Autodesk Inventor part; units mm, degrees
ref_plane "YZ Plane" through (0, 0, 0) normal (1, 0, 0) x (0, 1, 0)
ref_plane "XZ Plane" through (0, 0, 0) normal (0, 1, 0) x (-1, 0, 0)
ref_plane "XY Plane" through (0, 0, 0) normal (0, 0, 1) x (1, 0, 0)
sketch "Sketch1" plane through (0, 0, 0) normal (0, 0, 1) x (1, 0, 0)
  line L0 (-4.2, 0) -> (4.2, 0)
  line L1 (0, -1.5) -> (0, 9)
  line L2 (-3, 7.5) -> (3, 7.5)
  line L3 (3, 7.5) -> (3, 0)
  line L4 (3, 0) -> (-3, 0)
  line L5 (-3, 0) -> (-3, 7.5)
  point P0 (0, 0)
  point P1 (0, 0)
  dimension "d0" = 6
  dimension "d1" = 7.5
extrude "Extrusion1" add sketch "Sketch1" along normal mid plane 9.8
fillet "Fillet1" radius 3 2 edges at (3, 7.5, 0) (-3, 7.5, 0)
mirror "Mirror1" about plane through (-3, 0, 0) normal (0, -1, 0)
sketch "Sketch2" plane through (3, 4.5, 4.9) normal (1, 0, 0) x (0, 0, -1)
  point P0 (4.9, -4.5)
hole "Hole1" at (3, 0, 0) direction (-1, 0, 0) diameter 5 end through all
fillet "Fillet2" radius 2 2 edges at (3, 0, 2.5) (-3, 0, 2.5)
properties part number "P103" material "ABS Plastic"
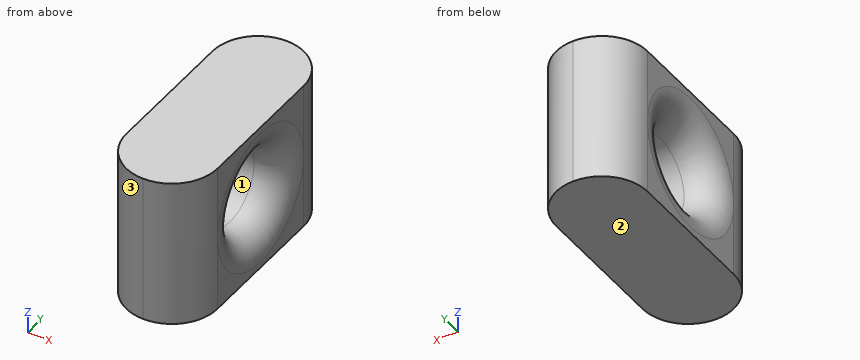
The model under review builds one solid part; all positions refer to its coordinate system, in mm. Face numbers are marked on the shaded views. Round coordinates to 2 decimals unless told otherwise and drop trailing zeros. Order: outer loops, then holes, each group sorted by start corner. A loop starts at its lowest first (then second) coordinate and runs counter-clockwise, first axis right, second up. Notation, with made-up numbers: M 23,19 L 43,19 A20 ccw 43,51 Z; hole C 65,80.25 d11. An arc over 180 degrees is marked long. Use a Markdown table: item, result.
1) Consider section C-C (x = -0.5). Write out the cut boundary in (y, z), then the cut area to 3 significant figures.
Report:
| item | result |
|---|---|
| outline | M -7.46,-4.9 L 7.46,-4.9 L 7.46,4.9 L -7.46,4.9 Z; hole C 0,0 d5 |
| area | 127 mm^2 |
2) Consider section B-B (y = 0). Write out the cut boundary in (x, z).
Report:
| item | result |
|---|---|
| outline | M -3,-4.9 L 3,-4.9 L 3,-4.5 A2 ccw 1,-2.5 L -1,-2.5 A2 ccw -3,-4.5 Z; M -3,4.5 A2 ccw -1,2.5 L 1,2.5 A2 ccw 3,4.5 L 3,4.9 L -3,4.9 Z |
3) Wall thickness on line 1 along Z through (x, y) = (-0.25, 0); line 2 along Y through (x, z) = (-0.4, 0); line 3 along Y through (x, z) = (-2.25, -0.25): over which ranges is each line inside the solid? List them lowest first. Write a range as [from, to].
Report:
| item | result |
|---|---|
| line 1 | [-4.9, -2.5], [2.5, 4.9] |
| line 2 | [-7.47, -2.5], [2.5, 7.47] |
| line 3 | [-6.48, -2.93], [2.93, 6.48] |
4) Consider section D-D (y = 6). Write out the cut boundary in (x, z), then the cut area to 3 significant figures.
Report:
| item | result |
|---|---|
| outline | M -2.6,-4.9 L 2.6,-4.9 L 2.6,4.9 L -2.6,4.9 Z |
| area | 50.9 mm^2 |
5) Draft analysis for pull direction Z (two halves, no side actions). For the marked faces 1, 2 and 3, state which applies: released by +Z, released by -Z, zero draft, split by the parting line, or undercut.
Report:
| item | result |
|---|---|
| face 1 | undercut |
| face 2 | released by -Z |
| face 3 | zero draft |
6) Insertion check: pin 1 (2 mm diameter, centred on y = -1.5, z = 2.5, fed in from -X). The pin has a flat end and moves straight along its axis. Give the tip position at first contact, or say it passes through.
Report:
| item | result |
|---|---|
| pin 1 | x = -2.91 |
